Autodesk Fusion 360 part; units mm, degrees
sketch "Sketch1" plane through (0, 0, 0) normal (0, 0, 1) x (1, 0, 0)
  line L0 (0, -2.5) -> (18.2, -2.5)
  arc A0 (18.2, -2.5) -> (18.2, 2.5) centre (18.2, 0) ccw
  line L1 (18.2, 2.5) -> (0, 2.5)
  arc A1 (0, 2.5) -> (0, -2.5) centre (0, 0) ccw
  line L2 (0, 0) -> (18.2, 0) construction
  circle A2 centre (0, 0) radius 0.9
  circle A3 centre (18.2, 0) radius 0.9
  dimension "d1" = 18.2
  dimension "d2" = 1.8
  dimension "d3" = 1.8
  dimension "d4" = 2.5
extrude "Extrude1" add sketch "Sketch1" along normal blind 2.5
For this review, take the finished solid that the model builds, in its own axes (mm). Coordinates: 2 decimals unless noted, no trailing zeros. Loops run counter-clockwise (first coordinate to the right, second up) from the corner with the lowest first, then second, coordinate; pieces in that order, holes last. Notation, with made-up numbers: (19, -1.75) -> (50, -1.75) arc R16 cw to (50, 2.25) -> close; hole circle Ø4 at (-1, -2.75). An arc over 180 degrees is marked (long way). Write each question's results on one line, items separated by ' | '.
Q1. Add section C-C, the plane y = 1.75. State the section outline as (x, z) points.
Taken from the geometry:
outline: (-1.79, 0) -> (19.99, 0) -> (19.99, 2.5) -> (-1.79, 2.5) -> close
Q2. Add section A-A, the plane y = 0. State the section outline as (x, z) points, then the cut area to 3 significant figures.
Taken from the geometry:
outline: (-2.5, 0) -> (-0.9, 0) -> (-0.9, 2.5) -> (-2.5, 2.5) -> close; (0.9, 0) -> (17.3, 0) -> (17.3, 2.5) -> (0.9, 2.5) -> close; (19.1, 0) -> (20.7, 0) -> (20.7, 2.5) -> (19.1, 2.5) -> close | area: 49.0 mm²
Q3. To check wall thickness, follow line 1 along Y through (x, z) = (18.2, 1.6); line 2 along X through (y, z) = (-1.5, 0.1); line 3 along X through (y, z) = (-2.25, 1.1). State the ranges of each line that lie inside material, in increasing order. Write a range as [from, to].
Taken from the geometry:
line 1: [-2.5, -0.9], [0.9, 2.5] | line 2: [-2, 20.2] | line 3: [-1.09, 19.29]
Q4. Mouldability with a two-part tool opening along X and no side actions: class faces 1 (the cylindrical face through (20.7, 0.1, 1.2)), 2 (the flat face through (9, -2.5, 1)), 3 (the cylindrical face through (19.06, -0.27, 1.23)) as +X half, -X half, draft (parallel to the pull), parting line (faces both ways), or undercut.
Taken from the geometry:
face 1: +X half | face 2: draft | face 3: undercut
Q5. Add section B-B, the plane z = 0.2. State the section outline as (x, y) points, then the cut area to 3 significant figures.
Taken from the geometry:
outline: (0, -2.5) -> (18.2, -2.5) arc R2.5 ccw to (18.2, 2.5) -> (0, 2.5) arc R2.5 ccw to start; hole circle Ø1.8 at (0, 0); hole circle Ø1.8 at (18.2, 0) | area: 106 mm²
